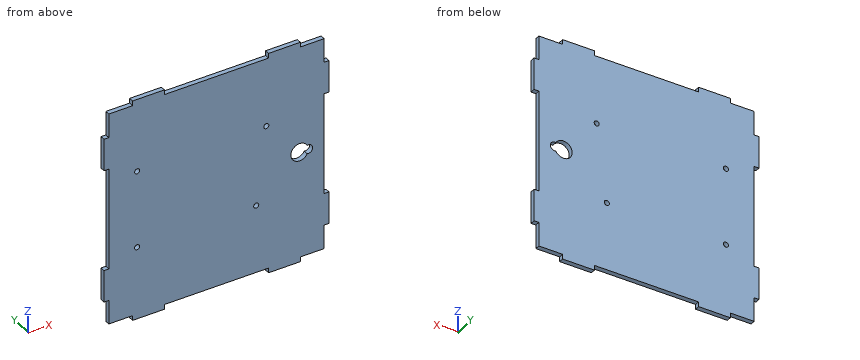
from build123d import *

# Parameters (mm, degrees)
SKETCH1_W           = 135.499999433
SKETCH1_H           = 133.500000387
BOSS_EXTRUDE1_DEPTH = 3
SKETCH2_W           = 3
SKETCH2_H           = 20
SKETCH2_W_2         = 20
SKETCH2_H_2         = 3
BOSS_EXTRUDE2_DEPTH = 3
SKETCH3_R           = 1.6
CUT_EXTRUDE1_DEPTH  = 115.913475286
SKETCH4_R           = 5.5
SKETCH4_R_2         = 2.75
CUT_EXTRUDE2_DEPTH  = 115.913475286


with BuildPart() as part:
    # Sketch1 → Boss-Extrude1 (new body)
    with BuildSketch(Plane(origin=(0, 0, 0), x_dir=(1, 0, 0), z_dir=(0, 1, 0))):
        with Locations((16.289033152, -5.21875036)):
            Rectangle(SKETCH1_W, SKETCH1_H)
    extrude(amount=BOSS_EXTRUDE1_DEPTH)

    # Sketch2 → Boss-Extrude2 (add, through all)
    with BuildSketch(Plane(origin=(0, 3, 0), x_dir=(1, 0, 0), z_dir=(0, 1, 0))):
        with Locations((85.539032868, 36.531249834)):
            Rectangle(SKETCH2_W, SKETCH2_H)
        with Locations((85.539032868, -46.968750553)):
            Rectangle(SKETCH2_W, SKETCH2_H)
        with Locations((59.039032868, 63.031249834)):
            Rectangle(SKETCH2_W_2, SKETCH2_H_2)
        with Locations((-26.460966565, 63.031249834)):
            Rectangle(SKETCH2_W_2, SKETCH2_H_2)
        with Locations((-52.960966565, 36.531249834)):
            Rectangle(SKETCH2_W, SKETCH2_H)
        with Locations((-52.960966565, -46.968750553)):
            Rectangle(SKETCH2_W, SKETCH2_H)
        with Locations((-26.460966565, -73.468750553)):
            Rectangle(SKETCH2_W_2, SKETCH2_H_2)
        with Locations((59.039032868, -73.468750553)):
            Rectangle(SKETCH2_W_2, SKETCH2_H_2)
    extrude(amount=-BOSS_EXTRUDE2_DEPTH)

    # Sketch3 → Cut-Extrude1 (cut, through all)
    with BuildSketch(Plane.XZ):
        with Locations(Location((-33.660968451, 29.22874915, 0), (0, 0, 270))):
            Circle(SKETCH3_R)
        with Locations(Location((47.619031549, 29.22874915, 0), (0, 0, 270))):
            Circle(SKETCH3_R)
        with Locations(Location((41.269031549, -19.03125085, 0), (0, 0, 270))):
            Circle(SKETCH3_R)
        with Locations(Location((-33.660968451, -19.03125085, 0), (0, 0, 270))):
            Circle(SKETCH3_R)
    extrude(amount=-CUT_EXTRUDE1_DEPTH, mode=Mode.SUBTRACT)

    # Sketch4 → Cut-Extrude2 (cut, through all)
    with BuildSketch(Plane.XZ):
        with Locations((68.539032868, 5.21875036)):
            Circle(SKETCH4_R)
        with Locations((74.039032868, 5.21875036)):
            Circle(SKETCH4_R_2)
    extrude(amount=-CUT_EXTRUDE2_DEPTH, mode=Mode.SUBTRACT)


solid = part.part
Model file for the job. Use its own axes, mm. Round coordinates to 2 decimals unless told otherwise and drop trailing zeros. Order: outer loops, then holes, each group sorted by start corner. A loop starts at its lowest first (then second) coordinate and runs counter-clockwise, first axis right, second up. Notation, with made-up numbers: M 5.5,75 L 60.5,75 A13 cw 60.5,86 Z; hole C 16,13.25 d4. An arc over 180 degrees is marked long. Write each question's results on one line, items separated by ' | '. Start each with the question number.
(1) Drop flat-ended pins along their axis: pin 1 (1 mm diameter, centred on x = -37, y = 2.5, fed in from +Z); pin 2 (1.5 mm diameter, centred on x = -44, y = 1, fed in from -Z); pin 3 (5 mm diameter, centred on x = -33.66, z = -19.03, fed in from -Y); pin 4 (1.5 mm diameter, centred on y = 2, z = 1, fed in from +X). Give the stop position or say it passes through.
(2) Saw through at C-C, the plane y = 2.55. State how many separate pieces and enclosed holes the cut face has, then the cut area to 3 significant figures.
(3) Probe probe 1 along X at (y, z) = (1.45, -18); probe 2 along X at (y, z) = (2.65, 30.5); probe 3 along X at (y, z) = (2.35, 26). List the from-to ranges inside material, lowest first. Write a range as from..to.
(4) Saw through at A-A, the plane x = 66.5. Give the cut face in (y, z).
(5) Saw through at D-D, the plane z = 24.5. Give the cut face in (x, y), then the cut area to 4 significant figures.
(6) Saw through at B-B, the plane x = 26. Give the cut face in (y, z), then the cut area to 4 significant figures.
Established:
1) pin 1: stops at z = 71.97 | pin 2: stops at z = -61.53 | pin 3: stops at y = 0 | pin 4: stops at x = 84.04
2) separate pieces: 1 | enclosed holes: 5 | area: 18,400 mm^2
3) probe 1: x = -51.46..-34.88, -32.44..40.05, 42.49..84.04 | probe 2: x = -51.46..-34.63, -32.69..46.65, 48.59..84.04 | probe 3: x = -51.46..84.04
4) outline: M 0,-64.53 L 3,-64.53 L 3,0.11 L 0,0.11 Z; M 0,10.33 L 3,10.33 L 3,74.97 L 0,74.97 Z
5) outline: M -51.46,0 L 84.04,0 L 84.04,3 L -51.46,3 Z | area: 406.5 mm^2
6) outline: M 0,-61.53 L 3,-61.53 L 3,71.97 L 0,71.97 Z | area: 400.5 mm^2
